Design review of the part built by this model. Coordinates are the model's own, in mm. Face numbers are marked on the shaded views. A direction names the side the tool comes from. Coordinates: 2 decimals unless noted, no trailing zeros. Order: outer loops, then holes, each group sorted by start corner. A loop starts at its lowest first (then second) coordinate and runs counter-clockwise, first axis right, second up. Notation, with made-up numbers: M -4,51.5 L 44,51.5 A16 cw 44,76.5 Z; hole C 78,79 d8. An arc over 180 degrees is marked long. Answer in a Markdown table with one row per item.
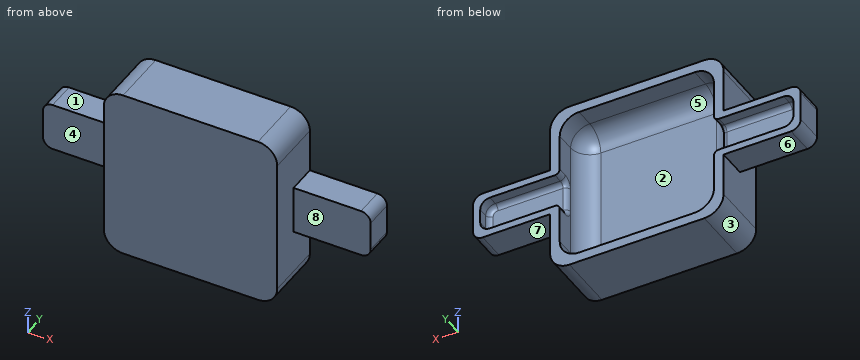
from build123d import *

# Parameters (mm, degrees)
BOSS_EXTRUDE1_DEPTH = 2
BOSS_EXTRUDE2_DEPTH = 4
FILLET1_R           = 2
BOSS_EXTRUDE3_DEPTH = 3
CUT_EXTRUDE1_DEPTH  = 1.5
FILLET2_R           = 0.5


with BuildPart() as part:
    # Sketch1 → Boss-Extrude1 (new body)
    with BuildSketch(Plane(origin=(0, 0, 0), x_dir=(1, 0, 0), z_dir=(0, 1, 0))):
        with BuildLine():
            Line((-7, -9), (7, -9))
            ThreePointArc((7, -9), (8.414213562, -8.414213562), (9, -7))
            Line((9, -7), (9, 7))
            ThreePointArc((9, 7), (8.414213562, 8.414213562), (7, 9))
            Line((7, 9), (-7, 9))
            ThreePointArc((-7, 9), (-8.414213562, 8.414213562), (-9, 7))
            Line((-9, 7), (-9, -7))
            ThreePointArc((-9, -7), (-8.414213562, -8.414213562), (-7, -9))
        make_face()
    extrude(amount=BOSS_EXTRUDE1_DEPTH)

    # Sketch2 → Boss-Extrude2 (add)
    with BuildSketch(Plane(origin=(0, 2, 0), x_dir=(1, 0, 0), z_dir=(0, 1, 0))):
        with BuildLine():
            Line((-7, -9), (7, -9))
            ThreePointArc((7, -9), (8.414213562, -8.414213562), (9, -7))
            Line((9, -7), (9, 7))
            ThreePointArc((9, 7), (8.414213562, 8.414213562), (7, 9))
            Line((7, 9), (-7, 9))
            ThreePointArc((-7, 9), (-8.414213562, 8.414213562), (-9, 7))
            Line((-9, 7), (-9, -7))
            ThreePointArc((-9, -7), (-8.414213562, -8.414213562), (-7, -9))
        make_face()
        with BuildLine():
            Line((-6, -8), (6, -8))
            ThreePointArc((6, -8), (7.414213562, -7.414213562), (8, -6))
            Line((8, -6), (8, 6))
            ThreePointArc((8, 6), (7.414213562, 7.414213562), (6, 8))
            Line((6, 8), (-6, 8))
            ThreePointArc((-6, 8), (-7.414213562, 7.414213562), (-8, 6))
            Line((-8, 6), (-8, -6))
            ThreePointArc((-8, -6), (-7.414213562, -7.414213562), (-6, -8))
        make_face(mode=Mode.SUBTRACT)
    extrude(amount=BOSS_EXTRUDE2_DEPTH)

    # Fillet1
    fillet1_edges = [part.edges().sort_by_distance(p)[0] for p in [
        (-7.414213562, 2, 7.414213562),
        (0, 2, 8),
        (7.414213562, 2, 7.414213562),
        (8, 2, 0),
        (7.414213562, 2, -7.414213562),
        (0, 2, -8),
        (-7.414213562, 2, -7.414213562),
        (-8, 2, 0),
    ]]
    fillet(fillet1_edges, radius=FILLET1_R)

    # Sketch3 → Boss-Extrude3 (add)
    with BuildSketch(Plane(origin=(0, 6, 0), x_dir=(1, 0, 0), z_dir=(0, 1, 0))):
        with BuildLine():
            Line((-9, 2.5), (-16, 2.5))
            ThreePointArc((-16, 2.5), (-16.707106781, 2.207106781), (-17, 1.5))
            Line((-17, 1.5), (-17, -1.5))
            ThreePointArc((-17, -1.5), (-16.707106781, -2.207106781), (-16, -2.5))
            Line((-16, -2.5), (-9, -2.5))
            Line((-9, -2.5), (-9, 2.5))
        make_face()
        with BuildLine():
            Line((9, 2.5), (16, 2.5))
            ThreePointArc((16, 2.5), (16.707106781, 2.207106781), (17, 1.5))
            Line((17, 1.5), (17, -1.5))
            ThreePointArc((17, -1.5), (16.707106781, -2.207106781), (16, -2.5))
            Line((16, -2.5), (9, -2.5))
            Line((9, -2.5), (9, 2.5))
        make_face()
    extrude(amount=-BOSS_EXTRUDE3_DEPTH)

    # Sketch4 → Cut-Extrude1 (cut)
    with BuildSketch(Plane(origin=(0, 6, 0), x_dir=(1, 0, 0), z_dir=(0, 1, 0))):
        with BuildLine():
            Line((-8, 1.75), (-15.25, 1.75))
            ThreePointArc((-15.25, 1.75), (-15.957106781, 1.457106781), (-16.25, 0.75))
            Line((-16.25, 0.75), (-16.25, -0.75))
            ThreePointArc((-16.25, -0.75), (-15.957106781, -1.457106781), (-15.25, -1.75))
            Line((-15.25, -1.75), (-8, -1.75))
            Line((-8, -1.75), (-8, 1.75))
        make_face()
        with BuildLine():
            Line((8, 1.75), (15.25, 1.75))
            ThreePointArc((15.25, 1.75), (15.957106781, 1.457106781), (16.25, 0.75))
            Line((16.25, 0.75), (16.25, -0.75))
            ThreePointArc((16.25, -0.75), (15.957106781, -1.457106781), (15.25, -1.75))
            Line((15.25, -1.75), (8, -1.75))
            Line((8, -1.75), (8, 1.75))
        make_face()
    extrude(amount=-CUT_EXTRUDE1_DEPTH, mode=Mode.SUBTRACT)

    # Fillet2
    fillet2_edges = [part.edges().sort_by_distance(p)[0] for p in [
        (-8, 4.5, 0),
        (-8, 5.25, -1.75),
        (-11.625, 4.5, 1.75),
        (-8, 5.25, 1.75),
        (-15.957106781, 4.5, 1.457106781),
        (-16.25, 4.5, 0),
        (-15.957106781, 4.5, -1.457106781),
        (-11.625, 4.5, -1.75),
        (8, 4.5, 0),
        (8, 5.25, 1.75),
        (11.625, 4.5, -1.75),
        (8, 5.25, -1.75),
        (15.957106781, 4.5, -1.457106781),
        (16.25, 4.5, 0),
        (15.957106781, 4.5, 1.457106781),
        (11.625, 4.5, 1.75),
    ]]
    fillet(fillet2_edges, radius=FILLET2_R - 0.0001)  # a hair under: the kernel refuses the full size


solid = part.part
(1) Insertion check: pin 1 Ø2 at (y, z) = (2.5, 6.5) entering from +X; pin 2 Ø1 at (y, z) = (5, 2.5) entering from +X; pin 3 Ø1 at (y, z) = (3.5, -5) entering from -X. Each pin has a flat end and moves straight along its axis. Give the tip position at first contact, or say it passes through.
Return value:
| item | result |
|---|---|
| pin 1 | stops at x = 9 |
| pin 2 | stops at x = 16.87 |
| pin 3 | stops at x = -9 |
(2) Draft analysis for pull direction X (two halves, no side actions). For the marked faces 1, 2 and 3, state which applies: pulls with the +X half, pulls with the -X half, needs draft (parallel to the pull), parting line crosses it, or undercut.
Return value:
| item | result |
|---|---|
| face 1 | needs draft |
| face 2 | undercut |
| face 3 | pulls with the -X half |
(3) Add section C-C, the plane z = -4.25. Give the boundary of the cut face in (x, y).
Return value:
| item | result |
|---|---|
| outline | M -9,0 L 9,0 L 9,6 L 8,6 L 8,4 A2 cw 6,2 L -6,2 A2 cw -8,4 L -8,6 L -9,6 Z |
(4) Add section B-B, the plane x = 2. Give the boundary of the cut face in (y, z).
Return value:
| item | result |
|---|---|
| outline | M 0,-9 L 6,-9 L 6,-8 L 4,-8 A2 cw 2,-6 L 2,6 A2 cw 4,8 L 6,8 L 6,9 L 0,9 Z |
(5) For line 1 along Z through (x, y) = (-14, 5.75); line 2 along X through (y, z) = (4.7, -3.75); line 3 along X through (y, z) = (2.85, 3), list the stretches that pass through material, from the lowest coordinate up. Write a range as from..to.
Return value:
| item | result |
|---|---|
| line 1 | z = -2.5..-1.75, 1.75..2.5 |
| line 2 | x = -9..-8, 8..9 |
| line 3 | x = -9..-7.64, 7.64..9 |
(6) For the marked faces 4, 5, 6, 7 and 8, list the 3-axis set-ups (+Z, -Z, +X, -X, +Y, -Y) from which the entire face can be reached by the end or side of a thin tool; tool diameter is ignored.
Return value:
| item | result |
|---|---|
| face 4 | +Z, -Z, -X, -Y |
| face 5 | +Y |
| face 6 | -Z, -X, +Y, -Y |
| face 7 | -Z, +X, +Y, -Y |
| face 8 | +Z, -Z, +X, -Y |
(7) Add section A-A, the plane y = 2.4. Give the boundary of the cut face in (x, z), and give its area (3 significant figures).
Return value:
| item | result |
|---|---|
| outline | M -9,-7 A2 ccw -7,-9 L 7,-9 A2 ccw 9,-7 L 9,7 A2 ccw 7,9 L -7,9 A2 ccw -9,7 Z; hole M -7.2,-6 A1.2 ccw -6,-7.2 L 6,-7.2 A1.2 ccw 7.2,-6 L 7.2,6 A1.2 ccw 6,7.2 L -6,7.2 A1.2 ccw -7.2,6 Z |
| area | 114 mm2 |
